```python
from build123d import *

# Parameters (mm, degrees)
SKETCH2_W           = 80
SKETCH2_H           = 20
BOSS_EXTRUDE1_DEPTH = 30
SKETCH3_W           = 20
SKETCH3_H           = 14
CUT_EXTRUDE1_DEPTH  = 30
SKETCH4_R           = 12
CUT_EXTRUDE2_DEPTH  = 30
SKETCH5_R           = 1.5
CUT_EXTRUDE3_DEPTH  = 30
SKETCH6_R           = 1.5
CUT_EXTRUDE4_DEPTH  = 3


with BuildPart() as part:
    # Sketch2 → Boss-Extrude1 (new body)
    with BuildSketch(Plane(origin=(0, 0, 0), x_dir=(1, 0, 0), z_dir=(0, 1, 0))):
        Rectangle(SKETCH2_W, SKETCH2_H)
    extrude(amount=BOSS_EXTRUDE1_DEPTH)

    # Sketch3 → Cut-Extrude1 (cut)
    with BuildSketch(Plane.XY.offset(10)):
        with Locations((30, 7)):
            Rectangle(SKETCH3_W, SKETCH3_H)
        with Locations((-30, 7)):
            Rectangle(SKETCH3_W, SKETCH3_H)
    extrude(amount=-CUT_EXTRUDE1_DEPTH, mode=Mode.SUBTRACT)

    # Sketch4 → Cut-Extrude2 (cut)
    with BuildSketch(Plane.XY.offset(10)):
        with Locations((0, 14.84)):
            Circle(SKETCH4_R)
    extrude(amount=-CUT_EXTRUDE2_DEPTH, mode=Mode.SUBTRACT)

    # Sketch5 → Cut-Extrude3 (cut)
    with BuildSketch(Plane(origin=(0, 30, 0), x_dir=(1, 0, 0), z_dir=(0, 1, 0))):
        with Locations((-35, 5)):
            Circle(SKETCH5_R)
        with Locations((-35, -5)):
            Circle(SKETCH5_R)
        with Locations((35, -5)):
            Circle(SKETCH5_R)
        with Locations((35, 5)):
            Circle(SKETCH5_R)
    extrude(amount=-CUT_EXTRUDE3_DEPTH, mode=Mode.SUBTRACT)

    # Sketch6 → Cut-Extrude4 (cut)
    with BuildSketch(Plane(origin=(0, 30, 0), x_dir=(1, 0, 0), z_dir=(0, 1, 0))):
        with Locations((-11.1, 5.89)):
            Circle(SKETCH6_R)
        with Locations((11.1, -4.41)):
            Circle(SKETCH6_R)
    extrude(amount=-CUT_EXTRUDE4_DEPTH, mode=Mode.SUBTRACT)


solid = part.part
```
Can you work these out from the model? Positions are in its coordinate system, mm. A direction names the side the tool comes from. Coordinates: 2 decimals unless noted, no trailing zeros. Loops run counter-clockwise (first coordinate to the right, second up) from the corner with the lowest first, then second, coordinate; pieces in that order, holes last.
1) Imagine slicing it at B-B on y = 22. List the corners of the cut face in (x, z) for me.
2) Imagine slicing it at D-D on x = -35. List the corners of the cut face in (y, z) for me.
3) For pin 1 (4 mm diameter, centred on y = 3.5, z = 2, fed in from +X); pin 2 (5 mm diameter, centred on x = -23.5, y = 10, fed in from -Z); pin 3 (6 mm diameter, centred on x = -28.5, z = 3, fed in from -Y); pin 4 (0.9 mm diameter, centred on x = 11, z = 4, fed in from +Y), each with a flat end and sliding along its axis, tell me the tip position at first contact or that it passes through.
4) Which directions (+Z, -Z, +X, -X, +Y, -Y) give clear straight access to the entire face, cutting with the end or side of a thin tool? Please do faces 1 (the flat face through (11, 27, 4)), 2 (the flat face through (20, 7, 0)), 3 (the cylindrical face through (33.8, 22.1, -4.1)), 4 (the flat face through (-20, 7, 0)).
5) Imagine slicing it at C-C on z = 0.75. List the corners of the cut face in (x, y) for me.
6) Imagine slicing it at A-A on x = 0. List the corners of the cut face in (y, z) for me.
7) I need wall thicknesses on probe 1 along X at (y, z) = (28.25, 4.25); probe 2 along X at (y, z) = (23.5, -5); probe 3 along X at (y, z) = (18.5, -2.25). Which ranges of each line are inside material? Lowest first, please.
8) Thinking about a two-plate mould opening in Z: for faces 5 (the flat face through (-1, 28, -10)), 6 (the cylindrical face through (-36.2, 22.1, -4.1)), 7 (the flat face through (0, 0, 0)), which applies, pulls with the +Z half, pulls with the -Z half, needs draft (parallel to the pull), parting line crosses it, or undercut?
Completed:
1. outline: (-40, -10) - (-9.63, -10) - (-9.63, 10) - (-40, 10) - close; (9.63, -10) - (40, -10) - (40, 10) - (9.63, 10) - close; hole circle Ø3 at (-35, -5); hole circle Ø3 at (-35, 5); hole circle Ø3 at (35, -5); hole circle Ø3 at (35, 5)
2. outline: (14, -10) - (30, -10) - (30, -6.5) - (14, -6.5) - close; (14, -3.5) - (30, -3.5) - (30, 3.5) - (14, 3.5) - close; (14, 6.5) - (30, 6.5) - (30, 10) - (14, 10) - close
3. pin 1: stops at x = 20
3. pin 2: passes through
3. pin 3: stops at y = 14
3. pin 4: stops at y = 27
4. face 1: +Y
4. face 2: +Z, -Z, +X, -Y
4. face 3: +Y, -Y
4. face 4: +Z, -Z, -X, -Y
5. outline: (-40, 14) - (-20, 14) - (-20, 0) - (20, 0) - (20, 14) - (40, 14) - (40, 30) - (-40, 30) - close; hole circle Ø24 at (0, 14.84)
6. outline: (0, -10) - (2.84, -10) - (2.84, 10) - (0, 10) - close; (26.84, -10) - (30, -10) - (30, 10) - (26.84, 10) - close
7. probe 1: x = -40 to -36.3, -33.7 to 9.61, 12.59 to 33.7, 36.3 to 40
7. probe 2: x = -40 to -36.5, -33.5 to -8.31, 8.31 to 33.5, 36.5 to 40
7. probe 3: x = -40 to -11.43, 11.43 to 40
8. face 5: pulls with the -Z half
8. face 6: undercut
8. face 7: needs draft
